from build123d import *

# Parameters (mm, degrees)
SALIENTE_EXTRUIR1_DEPTH = 35
CROQUIS2_R              = 23.966278947
CROQUIS2_R_2            = 11.5
CORTAR_EXTRUIR1_DEPTH   = 15
CROQUIS3_R              = 27.659664681
CROQUIS3_R_2            = 11.5
CORTAR_EXTRUIR2_DEPTH   = 16
CROQUIS4_W              = 90.840335319
CROQUIS4_H              = 30.090909091
CORTAR_EXTRUIR3_DEPTH   = 33
CROQUIS5_R              = 10
CORTAR_EXTRUIR5_DEPTH   = 33
CROQUIS6_R              = 10
CORTAR_EXTRUIR6_DEPTH   = 33


with BuildPart() as part:
    # Croquis1 → Saliente-Extruir1 (new body)
    with BuildSketch(Plane(origin=(0, 0, 0), x_dir=(1, 0, 0), z_dir=(0, 1, 0))):
        with BuildLine():
            Line((54, -25), (-39, -25))
            ThreePointArc((-39, -25), (-39.707106781, -24.707106781), (-40, -24))
            Line((-40, -24), (-40, -23.954545455))
            ThreePointArc((-40, -23.954545455), (-40.292893219, -23.247438673), (-41, -22.954545455))
            Line((-41, -22.954545455), (-54, -22.954545455))
            ThreePointArc((-54, -22.954545455), (-54.707106781, -22.661652236), (-55, -21.954545455))
            Line((-55, -21.954545455), (-55, 6.045454545))
            ThreePointArc((-55, 6.045454545), (-54.707106781, 6.752561327), (-54, 7.045454545))
            Line((-54, 7.045454545), (-41, 7.045454545))
            ThreePointArc((-41, 7.045454545), (-40.292893219, 7.338347764), (-40, 8.045454545))
            Line((-40, 8.045454545), (-40, 8.090909091))
            ThreePointArc((-40, 8.090909091), (-39.707106781, 8.798015872), (-39, 9.090909091))
            Line((-39, 9.090909091), (19, 9.090909091))
            ThreePointArc((19, 9.090909091), (19.707106781, 9.38380231), (20, 10.090909091))
            Line((20, 10.090909091), (20, 24))
            ThreePointArc((20, 24), (20.292893219, 24.707106781), (21, 25))
            Line((21, 25), (49, 25))
            ThreePointArc((49, 25), (49.707106781, 24.707106781), (50, 24))
            Line((50, 24), (50, 10.090909091))
            ThreePointArc((50, 10.090909091), (50.292893219, 9.38380231), (51, 9.090909091))
            Line((51, 9.090909091), (54, 9.090909091))
            ThreePointArc((54, 9.090909091), (54.707106781, 8.798015872), (55, 8.090909091))
            Line((55, 8.090909091), (55, -24))
            ThreePointArc((55, -24), (54.707106781, -24.707106781), (54, -25))
        make_face()
    extrude(amount=SALIENTE_EXTRUIR1_DEPTH)

    # Croquis2 → Cortar-Extruir1 (cut)
    with BuildSketch(Plane.ZY.offset(55)):
        with Locations((7.954545455, 17.5)):
            Circle(CROQUIS2_R)
        with Locations((7.954545455, 17.5)):
            Circle(CROQUIS2_R_2, mode=Mode.SUBTRACT)
    extrude(amount=-CORTAR_EXTRUIR1_DEPTH, mode=Mode.SUBTRACT)

    # Croquis3 → Cortar-Extruir2 (cut)
    with BuildSketch(Plane(origin=(0, 0, -25), x_dir=(-1, 0, 0), z_dir=(0, 0, -1))):
        with Locations((-35, 17.5)):
            Circle(CROQUIS3_R)
        with Locations((-35, 17.5)):
            Circle(CROQUIS3_R_2, mode=Mode.SUBTRACT)
    extrude(amount=-CORTAR_EXTRUIR2_DEPTH, mode=Mode.SUBTRACT)

    # Croquis4 → Cortar-Extruir3 (cut)
    with BuildSketch(Plane(origin=(0, 35, 0), x_dir=(1, 0, 0), z_dir=(0, 1, 0))):
        with Locations((7.42016766, -7.954545454)):
            Rectangle(CROQUIS4_W, CROQUIS4_H)
    extrude(amount=-CORTAR_EXTRUIR3_DEPTH, mode=Mode.SUBTRACT)

    # Croquis5 → Cortar-Extruir5 (cut)
    with BuildSketch(Plane.ZY.offset(55)):
        with Locations((7.954545455, 17.5)):
            Circle(CROQUIS5_R)
    extrude(amount=-CORTAR_EXTRUIR5_DEPTH, mode=Mode.SUBTRACT)

    # Croquis6 → Cortar-Extruir6 (cut)
    with BuildSketch(Plane(origin=(0, 0, -25), x_dir=(-1, 0, 0), z_dir=(0, 0, -1))):
        with Locations((-35, 17.5)):
            Circle(CROQUIS6_R)
    extrude(amount=-CORTAR_EXTRUIR6_DEPTH, mode=Mode.SUBTRACT)


solid = part.part
Verification items for the finished model (mm, model axes). A direction names the side the tool comes from. Coordinates: 2 decimals unless noted, no trailing zeros. Loops run counter-clockwise (first coordinate to the right, second up) from the corner with the lowest first, then second, coordinate; pieces in that order, holes last. Notation, with made-up numbers: M -28.75,-6.5 L 25.25,-6.5 A22 cw 25.25,10.5 Z; hole C 3,-1 d10. An arc over 180 degrees is marked long. One line per item, written item: value.
1. Set-up check for faces 4 (the flat face through (-40, 13, 19)), 5 (the flat face through (7, 19, -7.091)), 6 (the flat face through (26, 12, -25)), 7 (the flat face through (-13, 17, -9.091)), 8 (the flat face through (26, 10, -9)): record each of +Z, -Z, +X, -X, +Y, -Y from which the full face is reachable in a straight line by a thin tool's end or side.
Answers follow:
face 4: -X
face 5: +Y
face 6: -Z, +X, -X, +Y, -Y
face 7: -Z, -X, +Y, -Y
face 8: -Z
2. Mould release check, pull along X, two halves, no side actions. Record for faces 1 (the cylindrical face through (43.48, 25.27, -17.11)), 2 (the flat face through (-38, 26, 15)), 3 (the flat face through (8, 35, 24)): pulls with the +X half, pulls with the -X half, needs draft (parallel to the pull), parting line crosses it, or undercut.
Answers follow:
face 1: parting line crosses it
face 2: undercut
face 3: needs draft
3. Gauge pin test, flat ends, axial feed: P1, Ø9.5, axis at y = 20.5, z = 10, coming from the -X side; P2, Ø10, axis at x = 24.5, y = 12, coming from the -Z side; P3, Ø15, axis at x = 9, z = 9.5, coming from the +Y side; P4, Ø10, axis at y = 29.5, z = -15.5, coming from the -X side. Record the tip position at first contact, or that the pin passes through.
Answers follow:
P1: x = 52.84
P2: z = -25
P3: y = 2
P4: x = 25.88
4. Material ranges on line 1 along Z through (x, y) = (-25, 11.5); line 2 along X through (y, z) = (34.5, 18); line 3 along X through (y, z) = (26.5, 2), recorded low to high. Write a range as from..to.
Answers follow:
line 1: -9.09..-7.09, 23..25
line 2: -40..-38, 52.84..55
line 3: -55..-38, 52.84..55
5. Section check A-A on x = 35. Record the cut outline in (y, z).
Answers follow:
outline: M 0,-9 L 6,-9 L 6,-25 L 7.5,-25 L 7.5,-7.09 L 2,-7.09 L 2,23 L 35,23 L 35,25 L 0,25 Z; M 27.5,-25 L 29,-25 L 29,-9 L 35,-9 L 35,-7.09 L 27.5,-7.09 Z
6. Section check C-C on z = 1.5. Record the cut outline in (x, y).
Answers follow:
outline: M -55,7.98 L -40,7.98 L -40,0 L 55,0 L 55,35 L 52.84,35 L 52.84,2 L -38,2 L -38,9.86 L -55,9.86 Z; M -55,25.14 L -38,25.14 L -38,35 L -40,35 L -40,27.02 L -55,27.02 Z
7. Section check D-D on z = 20.5. Record the cut outline in (x, y), plus the area to 3 significant figures.
Answers follow:
outline: M -40,0 L 55,0 L 55,35 L 52.84,35 L 52.84,2 L -38,2 L -38,35 L -40,35 Z
area: 327 mm^2
